```python
from build123d import *

# Parameters (mm, degrees)
F0_R     = 4.213331
F0_R_2   = 5.128529
F0_R_3   = 3.464696
F0_R_4   = 1.5875
F0_R_5   = 3.175
F1_DEPTH = 3.048


with BuildPart() as f1:
    # F0 (on Front) → F1 (new body)
    with BuildSketch(Plane.XZ):
        with BuildLine():
            Line((2.690542, 12.411728), (0, 12.7))
            ThreePointArc((0, 12.7), (-8.980256, 8.980256), (-12.7, 0))
            ThreePointArc((-12.7, 0), (-8.980256, -8.980256), (0, -12.7))
            Line((0, -12.7), (2.690542, -12.411728))
            ThreePointArc((2.690542, -12.411728), (12.7, 0), (2.690542, 12.411728))
        make_face()
        Circle(F0_R, mode=Mode.SUBTRACT)
        with BuildLine():
            ThreePointArc((-12.7, 0), (-8.980256, 8.980256), (0, 12.7))
            Line((0, 12.7), (2.690542, 12.411728))
            ThreePointArc((2.690542, 12.411728), (12.7, 0), (2.690542, -12.411728))
            Line((2.690542, -12.411728), (44.45, -7.9375))
            ThreePointArc((44.45, -7.9375), (36.5125, 0), (44.45, 7.9375))
            Line((44.45, 7.9375), (20.738262, 10.478043))
            ThreePointArc((20.738262, 10.478043), (15.540023, 13.219546), (13.645066, 18.782519))
            Line((13.645066, 18.782519), (15.854942, 62.702238))
            ThreePointArc((15.854942, 62.702238), (0, 47.625), (-15.854942, 62.702238))
            Line((-15.854942, 62.702238), (-12.7, 0))
        make_face()
        with BuildLine():
            Line((2.690542, -12.411728), (0, -12.7))
            ThreePointArc((0, -12.7), (1.352971, -12.627726), (2.690542, -12.411728))
        make_face()
        with BuildLine():
            ThreePointArc((-15.854942, 64.297762), (-15.875, 63.5), (-15.854942, 62.702238))
            ThreePointArc((-15.854942, 62.702238), (0, 47.625), (15.854942, 62.702238))
            ThreePointArc((15.854942, 62.702238), (15.869985, 63.100993), (15.875, 63.5))
            ThreePointArc((15.875, 63.5), (15.869985, 63.899007), (15.854942, 64.297762))
            Line((15.854942, 64.297762), (15.553577, 66.678343))
            ThreePointArc((15.553577, 66.678343), (-0.023207, 79.374983), (-15.562803, 66.632855))
            Line((-15.562803, 66.632855), (-15.854942, 64.297762))
        make_face()
        with Locations((0, 63.5)):
            Circle(F0_R_2, mode=Mode.SUBTRACT)
        with BuildLine():
            ThreePointArc((-15.562803, 66.632855), (-15.752201, 65.470729), (-15.854942, 64.297762))
            Line((-15.854942, 64.297762), (-15.562803, 66.632855))
        make_face()
        with BuildLine():
            ThreePointArc((44.45, 7.9375), (36.5125, 0), (44.45, -7.9375))
            ThreePointArc((44.45, -7.9375), (50.06266, -5.61266), (52.3875, 0))
            ThreePointArc((52.3875, 0), (50.06266, 5.61266), (44.45, 7.9375))
        make_face()
        with Locations((44.45, 0)):
            Circle(F0_R_3, mode=Mode.SUBTRACT)
        with BuildLine():
            Line((-9.451321, 115.482438), (-15.562803, 66.632855))
            ThreePointArc((-15.562803, 66.632855), (-0.023207, 79.374983), (15.553577, 66.678343))
            Line((15.553577, 66.678343), (9.525, 114.3))
            ThreePointArc((9.525, 114.3), (-0.592365, 104.793438), (-9.451321, 115.482438))
        make_face()
        with Locations((-4.803868, 100.0252)):
            Circle(F0_R_4, mode=Mode.SUBTRACT)
        with BuildLine():
            ThreePointArc((15.854942, 64.297762), (15.749304, 65.493754), (15.553577, 66.678343))
            Line((15.553577, 66.678343), (15.854942, 64.297762))
        make_face()
        with BuildLine():
            ThreePointArc((9.525, 114.3), (0.592365, 123.806562), (-9.451321, 115.482438))
            ThreePointArc((-9.451321, 115.482438), (-0.592365, 104.793438), (9.525, 114.3))
        make_face()
        with Locations((0, 114.3)):
            Circle(F0_R_5, mode=Mode.SUBTRACT)
    extrude(amount=F1_DEPTH)


solid = f1.part
```
Design review of the part built by this model. Coordinates are the model's own, in mm. A direction names the side the tool comes from. Give positions to 0.01 mm unless a question says otherwise; leave off trailing zeros. Loops run counter-clockwise (first coordinate to the right, second up) from the corner with the lowest first, then second, coordinate; pieces in that order, holes last. Notation, with made-up numbers: (67, 13) -> (113, 13) arc R35 cw to (113, 49) -> close; hole circle Ø11 at (-27, -12). An arc over 180 degrees is marked (long way). One line per item, written item: value.
Q1. We need section D-D on x = 28. Give the boundary of the cut face in (y, z).
Numbers:
outline: (-3.05, -9.7) -> (0, -9.7) -> (0, 9.7) -> (-3.05, 9.7) -> close
Q2. Draft analysis for pull direction X (two halves, no side actions). For faces 1 (the cylindrical face through (-15.75, -1.5, 65.49)), 2 (the flat face through (3, -3.048, 41)), 3 (the cylindrical face through (-0.548, -1.503, 4.177)), state which applies: pulls with the +X half, pulls with the -X half, needs draft (parallel to the pull), parting line crosses it, or undercut.
Numbers:
face 1: pulls with the -X half
face 2: needs draft
face 3: undercut
Q3. Machinability: for faces 4 (the flat face through (14.735, -1.503, 40.435)), 5 (the flat face through (23.278, -1.503, -10.206)), which of the approach directions +Z, -Z, +X, -X, +Y, -Y give a long, thin tool a straight path to every point of the face, cutting with its end or side? Answer none if there is none.
Numbers:
face 4: +X, +Y, -Y
face 5: -Z, +X, +Y, -Y
Q4. We need section C-C on z = 73. Give the boundary of the cut face in (x, y), and give its area (3 significant figures).
Numbers:
outline: (-14.77, -3.05) -> (14.75, -3.05) -> (14.75, 0) -> (-14.77, 0) -> close
area: 90.0 mm^2
Q5. We need section A-A on y = -1.4. Give the number of separate pieces and of enclosed holes in the cut face, and give its area (3 significant figures).
Numbers:
separate pieces: 1
enclosed holes: 5
area: 4,040 mm^2
Q6. For pin 1 Ø5 at (x, z) = (0, 114.3) entering from -Y; pin 2 Ø1.5 at (y, z) = (-1.5, 23) entering from -X (3 decimals); pin 3 Ø8 at (x, z) = (44.45, 0) entering from -Y; pin 4 Ø1 at (x, y) = (-1, -0.5) entering from +Z, all flat-tipped, find the tip position at first contact; note any pin that passes through.
Numbers:
pin 1: passes through
pin 2: stops at x = -13.895
pin 3: stops at y = -3.05
pin 4: stops at z = 123.81
Q7. We need section B-B on x = 46.5. Give the boundary of the cut face in (y, z).
Numbers:
outline: (-3.05, -7.67) -> (0, -7.67) -> (0, -2.79) -> (-3.05, -2.79) -> close; (-3.05, 2.79) -> (0, 2.79) -> (0, 7.67) -> (-3.05, 7.67) -> close
Q8. For L1, parallel to Z at x = 0, y = -1.9 (3 decimals); L2, parallel to Z at x = -2.5, y = -2.3; L3, parallel to Z at x = 45.5, y = -1.8, list the stretches that pass through material, from the lowest coordinate up.
Numbers:
L1: z = -12.7 to -4.213, 4.213 to 58.371, 68.629 to 111.125, 117.475 to 123.825
L2: z = -12.45 to -3.39, 3.39 to 59.02, 67.98 to 112.34, 116.26 to 123.49
L3: z = -7.87 to -3.3, 3.3 to 7.87
